```python
from build123d import *

# Parameters (mm, degrees)
SKETCH1_R           = 1.7145
BOSS_EXTRUDE1_DEPTH = 127


with BuildPart() as part:
    # Sketch1 → Boss-Extrude1 (new, symmetric)
    with BuildSketch(Plane.XY):
        Polygon((6.35, 0), (3.175, 5.499261314), (-3.175, 5.499261314), (-6.35, 0), (-3.175, -5.499261314), (3.175, -5.499261314), align=None)
        Circle(SKETCH1_R, mode=Mode.SUBTRACT)
    extrude(amount=BOSS_EXTRUDE1_DEPTH, both=True)


solid = part.part
```
Model file for the job. Use its own axes, mm. Give positions to 0.01 mm unless a question says otherwise; leave off trailing zeros. Order: outer loops, then holes, each group sorted by start corner. A loop starts at its lowest first (then second) coordinate and runs counter-clockwise, first axis right, second up.
1) Pin check, flat tips, straight feed: pin 1 (1 mm diameter, centred on y = 1, z = 34, fed in from +X); pin 2 (1 mm diameter, centred on y = -4, z = 24, fed in from +X); pin 3 (1.5 mm diameter, centred on y = -4, z = -37.5, fed in from -X); pin 4 (2.5 mm diameter, centred on x = 0, y = 0, fed in from -Z). Stop position of each tip, or through.
2) Saw through at B-B, the plane y = -3.5. Write the cut outline in (x, z), then the cut area to 3 significant figures.
3) Wall check: probe 1 along Y at (x, z) = (-0.25, -17.5); probe 2 along X at (y, z) = (0.5, 73.5); probe 3 along X at (y, z) = (-1.5, -44.5). Give the ranges that are in metal, low to high.
Computed:
1. pin 1: stops at x = 6.06
1. pin 2: stops at x = 4.33
1. pin 3: stops at x = -4.47
1. pin 4: passes through
2. outline: (-4.33, -127) - (4.33, -127) - (4.33, 127) - (-4.33, 127) - close
2. area: 2,200 mm2
3. probe 1: y = -5.5 to -1.7, 1.7 to 5.5
3. probe 2: x = -6.06 to -1.64, 1.64 to 6.06
3. probe 3: x = -5.48 to -0.83, 0.83 to 5.48
